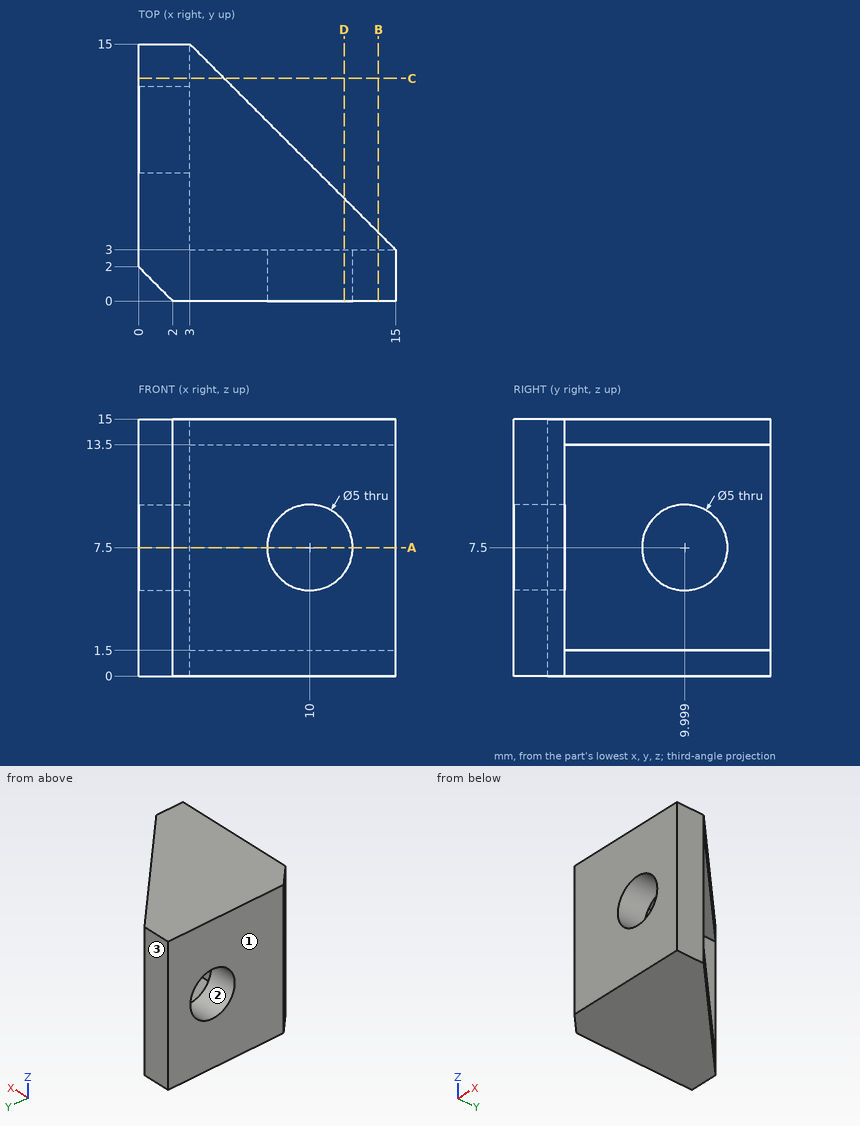
The figure shows three views and two pictorial views of one solid part (mm, origin at its lowest corner). Answer the questions. Give positions to 0.01 mm unless a question says otherwise; leave off trailing zeros. Loops run counter-clockwise (first coordinate to the right, second up) from the corner with the lowest first, then second, coordinate; pieces in that order, holes last. Notation, with made-up numbers: (17, 2) -> (56, 2) arc R31 ccw to (56, 35) -> close; hole circle Ø9 at (59, 12.5). An arc over 180 degrees is marked (long way). Use a Markdown table: item, result. Add a question column.
1. Section C-C on y = 13 is taken. Determine the outline of the cut face in (x, z).
2. Section B-B on x = 14 is taken. Determine the outline of the cut face in (y, z).
3. Section A-A on z = 7.5 is taken. Determine the outline of the cut face in (x, y).
4. Determine the mould class of the marked faces 1, 2 and 3 for opening direction Y: released by +Y, released by -Y, zero draft, split by the parting line, or undercut.
5. Find the intervals of material crossed by probe 1 along Z at (x, y) = (8.5, 6.5); probe 2 along X at (y, z) = (7.5, 3.5), in increasing order.
6. Section D-D on x = 12 is taken. Determine the outline of the cut face in (y, z).
7. Flat-ended cylindrical pins translate along their axes: pin 1 Ø4 at (x, z) = (12.5, 5.5) entering from -Y; pin 2 Ø3.5 at (x, z) = (10, 9) entering from +Y; pin 3 Ø8 at (y, z) = (9.999, 7.5) entering from +X. Find the tip coordinate at first contact, or state that the pin passes through.
Results below:
| question | item | result |
|---|---|---|
| 1 | outline | (0, 0) -> (5, 0) -> (5, 1.5) -> (3, 1.5) -> (3, 13.5) -> (5, 13.5) -> (5, 15) -> (0, 15) -> close |
| 2 | outline | (0, 0) -> (4, 0) -> (4, 1.5) -> (3, 1.5) -> (3, 13.5) -> (4, 13.5) -> (4, 15) -> (0, 15) -> close |
| 3 | outline | (0, 2) -> (2, 0) -> (7.5, 0) -> (7.5, 3) -> (3, 3) -> (3, 7.5) -> (0, 7.5) -> close; (0, 12.5) -> (3, 12.5) -> (3, 15) -> (0, 15) -> close; (12.5, 0) -> (15, 0) -> (15, 3) -> (12.5, 3) -> close |
| 4 | face 1 | zero draft |
| 4 | face 2 | undercut |
| 4 | face 3 | released by +Y |
| 5 | probe 1 | z = 0 to 1.5, 13.5 to 15 |
| 5 | probe 2 | x = 0 to 3 |
| 6 | outline | (0, 0) -> (6, 0) -> (6, 1.5) -> (3, 1.5) -> (3, 6) -> (0, 6) -> close; (0, 9) -> (3, 9) -> (3, 13.5) -> (6, 13.5) -> (6, 15) -> (0, 15) -> close |
| 7 | pin 1 | stops at y = 0 |
| 7 | pin 2 | stops at y = 3 |
| 7 | pin 3 | stops at x = 3 |
